Part print with two shaded views. Sizes in mm from the minimum x, y, z corner. Round coordinates to 2 decimals unless told otherwise and drop trailing zeros. Loops run counter-clockwise (first coordinate to the right, second up) from the corner with the lowest first, then second, coordinate; pieces in that order, holes last.
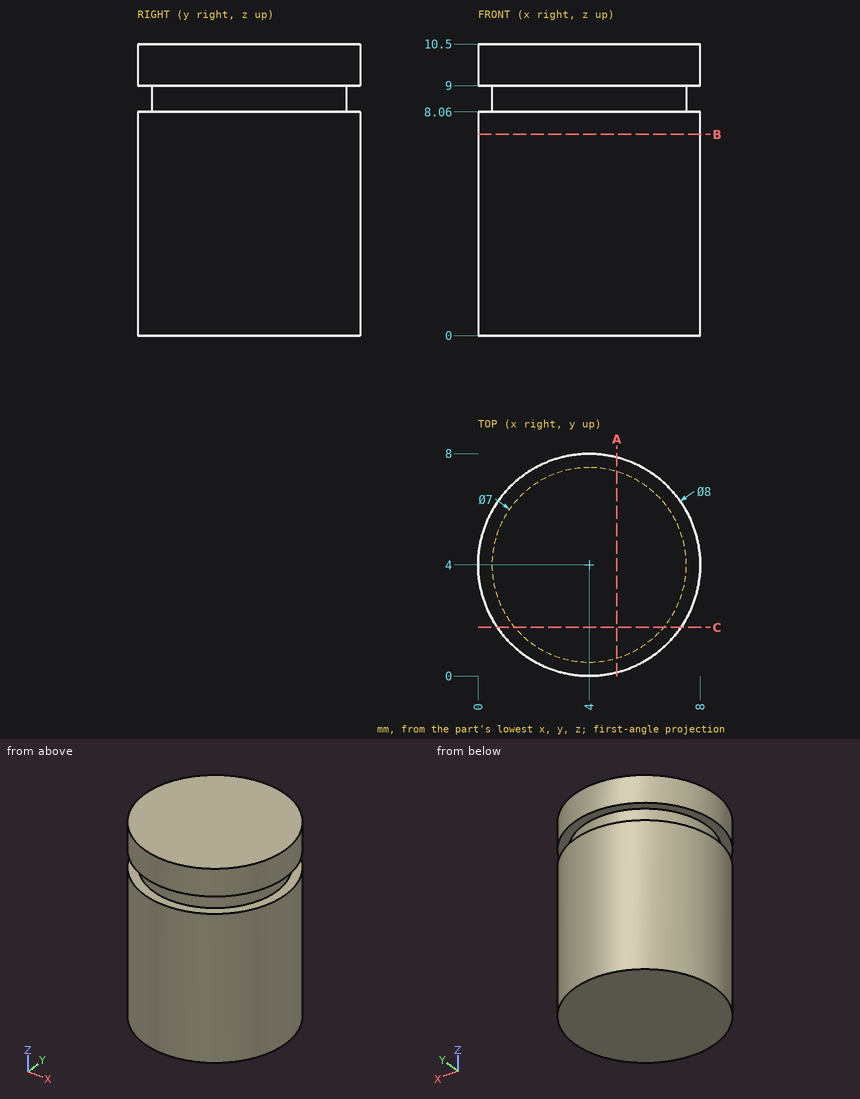
Item 1: Wall check: L1, parallel to Z at x = 2.5, y = 0.5; L2, parallel to X at y = 2.5, z = 4.5; L3, parallel to Y at x = 1.75, z = 3.25. Give the ranges that are in metal, low to high.
Verdict:
L1: z = 0 to 8.06, 9 to 10.5
L2: x = 0.29 to 7.71
L3: y = 0.69 to 7.31
Item 2: Cut at A-A (x = 5). List the corners of the cut face in (y, z), plus the area to 3 significant figures.
Verdict:
outline: (0.13, 0) - (7.87, 0) - (7.87, 8.06) - (7.35, 8.06) - (7.35, 9) - (7.87, 9) - (7.87, 10.5) - (0.13, 10.5) - (0.13, 9) - (0.65, 9) - (0.65, 8.06) - (0.13, 8.06) - close
area: 80.4 mm2
Item 3: Cut at C-C (y = 1.75). List the corners of the cut face in (x, z).
Verdict:
outline: (0.69, 0) - (7.31, 0) - (7.31, 8.06) - (6.68, 8.06) - (6.68, 9) - (7.31, 9) - (7.31, 10.5) - (0.69, 10.5) - (0.69, 9) - (1.32, 9) - (1.32, 8.06) - (0.69, 8.06) - close
Item 4: Cut at B-B (z = 7.25). List the corners of the cut face in (x, y), plus the area to 3 significant figures.
Verdict:
outline: circle Ø8 at (4, 4)
area: 50.3 mm2
Item 5: Flat gauge pins, fed straight in: P1, Ø4, axis at y = 6.5, z = 8, coming from the +X side; P2, Ø2, axis at x = 1.5, z = 2, coming from the -Y side; P3, Ø2, axis at y = 1, z = 6.5, coming from the -X side. Where does each tip first touch, or does it go through?
Verdict:
P1: stops at x = 7.97
P2: stops at y = 0.29
P3: stops at x = 0.54
